```python
from build123d import *

# Parameters (mm, degrees)
SKETCH_1_W          = 95
SKETCH_1_H          = 38.85
EXTRUDE_1_DEPTH     = 0.5
SKETCH_2_W          = 38.85
SKETCH_2_H          = 95
EXTRUDE_2_DEPTH     = 0.5
CUT_EXTRUDE_1_DEPTH = 110.347085009


with BuildPart() as part:
    # Эскиз1 → Бобышка-Вытянуть1 (new body)
    with BuildSketch(Plane(origin=(0.5, 0, 0), x_dir=(0, -1, 0), z_dir=(-1, 0, 0))):
        with Locations((-53.35, 22.825)):
            Rectangle(SKETCH_1_W, SKETCH_1_H)
    extrude(amount=-EXTRUDE_1_DEPTH)

    # Эскиз2 → Бобышка-Вытянуть2 (add)
    with BuildSketch(Plane.ZY.offset(-0.5)):
        with Locations((22.825, 53.35)):
            Rectangle(SKETCH_2_W, SKETCH_2_H)
    extrude(amount=EXTRUDE_2_DEPTH)

    # Эскиз3 → Вырез-Вытянуть1 (cut, through all)
    with BuildSketch(Plane.ZY):
        Polygon((-5.326732783, 46.541852111), (17.306560977, 46.5418531), (17.306560338, 61.155899742), (-5.326732783, 61.155898752), align=None)
    extrude(amount=-CUT_EXTRUDE_1_DEPTH, mode=Mode.SUBTRACT)


solid = part.part
```
Verification items for the finished model (mm, model axes). Round coordinates to 2 decimals unless told otherwise and drop trailing zeros. Write each loop counter-clockwise with the first axis right and the second up, starting at its lowest first coordinate (ties: lowest second). Pieces come first, ordered by that corner, then holes.
1. Section check A-A on z = 15.5. Enter the section's corners in (x, y), plus the area to 3 significant figures.
2. Section check C-C on y = 58.5. Enter the section's corners in (x, z).
3. Scan lines: L1, parallel to Y at x = 0.7, z = 8.5; L2, parallel to Z at x = 0.6, y = 51.5. Record each from-to range of solid material in increasing order.
4. Section check B-B on x = 0.3. Enter the section's corners in (y, z), plus the area to 3 significant figures.
Answer:
1. outline: (0, 5.85) - (1, 5.85) - (1, 46.54) - (0, 46.54) - close; (0, 61.16) - (1, 61.16) - (1, 100.85) - (0, 100.85) - close
1. area: 80.4 mm2
2. outline: (0, 17.31) - (1, 17.31) - (1, 42.25) - (0, 42.25) - close
3. L1: y = 5.85 to 46.54, 61.16 to 100.85
3. L2: z = 17.31 to 42.25
4. outline: (5.85, 3.4) - (46.54, 3.4) - (46.54, 17.31) - (61.16, 17.31) - (61.16, 3.4) - (100.85, 3.4) - (100.85, 42.25) - (5.85, 42.25) - close
4. area: 3,490 mm2
